Here's how the part is built. I have some questions about the finished solid (model axes, mm). A direction names the side the tool comes from. Coordinates: 2 decimals unless noted, no trailing zeros. Loops run counter-clockwise (first coordinate to the right, second up) from the corner with the lowest first, then second, coordinate; pieces in that order, holes last. Notation, with made-up numbers: (28.5, 56.5) -> (78.5, 56.5) arc R21 ccw to (78.5, 91.5) -> close; hole circle Ø10 at (-15, 17.25). An arc over 180 degrees is marked (long way). Answer as a JSON object with one key per item and string values. Group by question number.
Q1. I want a section at B-B on z = 6.5. Write out the boundary of the cut face in (x, y), then the cut area to 3 significant figures.
Q2. I'm going to push a flat-ended pin straight in: pin 1 (5 mm diameter, centred on y = -31.5, z = 7, fed in from -X). Where does the tip first touch, or does it pass through?
Q3. I want a section at A-A on x = 7. Write out the boundary of the cut face in (y, z).
Q4. I need wall thicknesses on line 1 (Z direction, x = 15, y = -31); line 2 (Y direction, x = 13.5, z = 1); line 3 (X direction, y = -31.5, z = -7). Which ranges of each line are inside material? Lowest first, please.
Q5. On a 3-axis mill with a long thin cutter (end or side, diameter ignored), from which of +Z, -Z, +X, -X, +Y, -Y can I reach the whole of each face in a straight line? I mean faces 5 (the flat face through (-1, 0, 0)), 6 (the flat face through (-1, -19, -0.5)). Say none if no direction works.
Q6. Thinking about a two-plate mould opening in Z: for faces 1 (the flat face through (-1, -19, -22)), 2 (the flat face through (-1, -19, 20.5)), 3 (the flat face through (-1, -1.5, -11)), 4 (the flat face through (-1, -39, 0)), which applies, released by +Z, released by -Z, zero draft, split by the parting line, or undercut?
Q7. I want a section at C-C on y = -11. Write out the boundary of the cut face in (x, z).
```python
from build123d import *

# Parameters (mm, degrees)
F0_W     = 110
F0_H     = 44
F1_DEPTH = 39
F2_W     = 36
F2_H     = 20
F3_DEPTH = 109


with BuildPart() as f1:
    # F0 (on Front) → F1 (new body)
    with BuildSketch(Plane.XZ):
        Rectangle(F0_W, F0_H)
    extrude(amount=F1_DEPTH)

    # F2 (on face) → F3 (cut)
    with BuildSketch(Plane(origin=(-55, 0, 0), x_dir=(0, -1, 0), z_dir=(-1, 0, 0))):
        with Locations((19.5, 10.5)):
            Rectangle(F2_W, F2_H)
        with Locations((19.5, -10.5)):
            Rectangle(F2_W, F2_H)
    extrude(amount=-F3_DEPTH, mode=Mode.SUBTRACT)


solid = f1.part
```
Result set:
{
 "1": {"outline": "(-55, -39) -> (55, -39) -> (55, 0) -> (-55, 0) -> (-55, -1.5) -> (54, -1.5) -> (54, -37.5) -> (-55, -37.5) -> close", "area": "366 mm²"},
 "2": {"pin 1": "stops at x = 54"},
 "3": {"outline": "(-39, -22) -> (0, -22) -> (0, 22) -> (-39, 22) -> close; hole (-37.5, -20.5) -> (-1.5, -20.5) -> (-1.5, -0.5) -> (-37.5, -0.5) -> close; hole (-37.5, 0.5) -> (-1.5, 0.5) -> (-1.5, 20.5) -> (-37.5, 20.5) -> close"},
 "4": {"line 1": "z = -22 to -20.5, -0.5 to 0.5, 20.5 to 22", "line 2": "y = -39 to -37.5, -1.5 to 0", "line 3": "x = 54 to 55"},
 "5": {"face 5": "+Z, -Z, +X, -X, +Y", "face 6": "-X"},
 "6": {"face 1": "released by -Z", "face 2": "undercut", "face 3": "undercut", "face 4": "zero draft"},
 "7": {"outline": "(-55, -22) -> (55, -22) -> (55, 22) -> (-55, 22) -> (-55, 20.5) -> (54, 20.5) -> (54, 0.5) -> (-55, 0.5) -> (-55, -0.5) -> (54, -0.5) -> (54, -20.5) -> (-55, -20.5) -> close"}
}
